from build123d import *

# Parameters (mm, degrees)
SKETCH1_R                = 143
SKETCH1_R_2              = 50
BOSS_EXTRUDE1_DEPTH      = 6.9
SKETCH2_R                = 1.85
BOSS_EXTRUDE2_DEPTH      = 6.9
FILLET1_R                = 30
CIRPATTERN1_COUNT        = 6
FILLET1_OF_CIRPATTERN1_R = 30
CUT_EXTRUDE1_DEPTH       = 214.214938645
FILLET3_R                = 5
CIRPATTERN2_COUNT        = 6
FILLET3_OF_CIRPATTERN2_R = 5
CUT_EXTRUDE2_DEPTH       = 10
FILLET4_R                = 10
FILLET5_START            = -1
FILLET5_DEPTH            = 9


with BuildPart() as part:
    # Sketch1 → Boss-Extrude1 (new body)
    with BuildSketch(Plane.XY):
        with Locations(Location((0, 0, 0), (0, 0, 180))):
            Circle(SKETCH1_R)
        with Locations(Location((0, 0, 0), (0, 0, 180))):
            Circle(SKETCH1_R_2, mode=Mode.SUBTRACT)
    extrude(amount=BOSS_EXTRUDE1_DEPTH)

    # Sketch2 → Boss-Extrude2 (add)
    with BuildSketch(Plane.XY.offset(6.9)):
        with BuildLine():
            Line((-136, -8), (-150, -8))
            ThreePointArc((-150, -8), (-158, 0), (-150, 8))
            Line((-150, 8), (-136, 8))
            ThreePointArc((-136, 8), (-128, 0), (-136, -8))
        make_face()
        with Locations((-150, 0)):
            Circle(SKETCH2_R, mode=Mode.SUBTRACT)
    boss_extrude2 = extrude(amount=-BOSS_EXTRUDE2_DEPTH)

    # Fillet1
    fillet1_edges = [part.edges().sort_by_distance(p)[0] for p in [
        (-142.776048411, 8, 3.45),
        (-142.776048411, -8, 3.45),
    ]]
    fillet(fillet1_edges, radius=FILLET1_R)

    # CirPattern1: Boss-Extrude2 ×6 about axis
    cirpattern1_axis = Axis((0, 0, 0), (0, 0, 1))
    for i in range(1, CIRPATTERN1_COUNT):
        add(boss_extrude2.rotate(cirpattern1_axis, i * 360 / CIRPATTERN1_COUNT))

    # Fillet1 of CirPattern1
    fillet1_of_cirpattern1_edges = [part.edges().sort_by_distance(p)[0] for p in [
        (-78.316227436, -119.647684976, 3.45),
        (-64.459820975, -127.647684976, 3.45),
        (64.459820975, -127.647684976, 3.45),
        (78.316227436, -119.647684976, 3.45),
        (142.776048411, -8, 3.45),
        (142.776048411, 8, 3.45),
        (78.316227436, 119.647684976, 3.45),
        (64.459820975, 127.647684976, 3.45),
        (-64.459820975, 127.647684976, 3.45),
        (-78.316227436, 119.647684976, 3.45),
    ]]
    fillet(fillet1_of_cirpattern1_edges, radius=FILLET1_OF_CIRPATTERN1_R)

    # Sketch7 → Cut-Extrude1 (cut, through all)
    with BuildSketch(Plane.XY.offset(6.9)):
        with BuildLine():
            Line((-30, 158), (30, 158))
            ThreePointArc((30, 158), (45, 143), (30, 128))
            Line((30, 128), (-30, 128))
            ThreePointArc((-30, 128), (-45, 143), (-30, 158))
        make_face()
    cut_extrude1 = extrude(amount=-CUT_EXTRUDE1_DEPTH, mode=Mode.SUBTRACT)

    # Fillet3
    fillet3_edges = [part.edges().sort_by_distance(p)[0] for p in [
        (43.398254251, 136.255610996, 3.45),
        (-43.398254251, 136.255610996, 3.45),
    ]]
    fillet(fillet3_edges, radius=FILLET3_R)

    # CirPattern2: Cut-Extrude1 ×6 about axis
    cirpattern2_axis = Axis((0, 0, 0), (0, 0, 1))
    for i in range(1, CIRPATTERN2_COUNT):
        add(cut_extrude1.rotate(cirpattern2_axis, i * 360 / CIRPATTERN2_COUNT), mode=Mode.SUBTRACT)

    # Fillet3 of CirPattern2
    fillet3_of_cirpattern2_edges = [part.edges().sort_by_distance(p)[0] for p in [
        (-96.301693406, 105.711796159, 3.45),
        (-139.699947656, 30.543814837, 3.45),
        (-139.699947656, -30.543814837, 3.45),
        (-96.301693406, -105.711796159, 3.45),
        (-43.398254251, -136.255610996, 3.45),
        (43.398254251, -136.255610996, 3.45),
        (96.301693406, -105.711796159, 3.45),
        (139.699947656, -30.543814837, 3.45),
        (139.699947656, 30.543814837, 3.45),
        (96.301693406, 105.711796159, 3.45),
    ]]
    fillet(fillet3_of_cirpattern2_edges, radius=FILLET3_OF_CIRPATTERN2_R)

    # Sketch8 → Cut-Extrude2 (cut)
    with BuildSketch(Plane.XY.offset(6.9)):
        with BuildLine():
            Line((88.826969439, -117.302003887), (84.326969439, -109.507775253))
            ThreePointArc((84.326969439, -109.507775253), (78.727650946, -108.125342861), (77.567379868, -113.774878941))
            Line((77.567379868, -113.774878941), (81.895896581, -121.29702529))
            ThreePointArc((81.895896581, -121.29702529), (87.360379041, -122.76754121), (88.826969439, -117.302003887))
        make_face()
        with BuildLine():
            Line((64.101233792, -131.577414018), (59.601233792, -123.783185384))
            ThreePointArc((59.601233792, -123.783185384), (54.136918717, -122.319207019), (52.673277073, -127.783612295))
            Line((52.673277073, -127.783612295), (57.221343973, -135.658853653))
            ThreePointArc((57.221343973, -135.658853653), (62.677994964, -137.017599926), (64.101233792, -131.577414018))
        make_face()
    extrude(amount=-CUT_EXTRUDE2_DEPTH, mode=Mode.SUBTRACT)

    # Fillet4
    fillet4_edges = [part.edges().sort_by_distance(p)[0] for p in [
        (64.565608345, -134.330457838, 3.45),
        (84.050784817, -123.080685956, 3.45),
    ]]
    fillet(fillet4_edges, radius=FILLET4_R)

    # Fillet5: read off the stored shape, not the designer's step
    # Fillet5 outline → Fillet5 (cut)
    with BuildSketch(Plane.XY.offset(FILLET5_START)):
        with BuildLine():
            ThreePointArc((87.553061033, -115.095529803), (90.213766815, -111.477504252), (93.384762884, -108.297213687))
            ThreePointArc((93.384762884, -108.297213687), (88.166794559, -109.665787745), (82.997135719, -108.124743986))
            ThreePointArc((82.997135719, -108.124743986), (83.746204288, -108.73534476), (84.326969439, -109.507775253))
            Line((84.326969439, -109.507775253), (87.553061033, -115.095529803))
        make_face()
        with BuildLine():
            ThreePointArc((52.14020721, -125.939999968), (50.889960833, -131.187577731), (47.09575677, -135.022183827))
            ThreePointArc((47.09575677, -135.022183827), (51.435909668, -133.866082974), (55.900021902, -133.370907928))
            Line((55.900021902, -133.370907928), (52.673277073, -127.783612295))
            ThreePointArc((52.673277073, -127.783612295), (52.294537166, -126.894249553), (52.14020721, -125.939999968))
        make_face()
    extrude(amount=FILLET5_DEPTH, mode=Mode.SUBTRACT)


solid = part.part
Build history of the part. All positions in model axes, mm. A direction names the side the tool comes from. Coordinates: 2 decimals unless noted, no trailing zeros. Order: outer loops, then holes, each group sorted by start corner. A loop starts at its lowest first (then second) coordinate and runs counter-clockwise, first axis right, second up. Notation, with made-up numbers: (4, 20) - (21, 20) arc R19 ccw to (21, 50) - close; hole circle Ø6 at (-34.5, 87). An arc over 180 degrees is marked (long way). Write each question's results on one line, items separated by ' | '. Start each with the question number.
Item 1: Band-saw the part on A-A on x = 0. Write the cut outline in (y, z).
Item 2: Mould opens along Y. For faces 4 (the face through (36.324, -129.398, 3.498)), 5 (the face through (-93.9, -96.16, 3.5)), 6 (the face through (2, 59, 0)) say: released by +Y, released by -Y, zero draft, split by the parting line, or undercut.
Item 3: Tool access for faces 1 (the face through (110.641, -64.364, 3.498)), 2 (the face through (36.492, 129.478, 3.498)), 3 (the face through (0, -128, 3)): list every direction of +Z, -Z, +X, -X, +Y, -Y with a clear straight run to the whole face (end or side of a thin tool).
Item 4: Flat gauge pins, fed straight in: pin 1 (1.5 mm diameter, centred on x = -56.5, z = 2.5, fed in from +Y); pin 2 (2 mm diameter, centred on x = -75, y = 129.9, fed in from +Z); pin 3 (3 mm diameter, centred on x = 59, z = 1.5, fed in from +Y); pin 4 (1.5 mm diameter, centred on x = -87, z = 2.5, fed in from -Y). Where does each tip first touch, or does it go through?
Item 5: Band-saw the part on C-C on y = -85. Write the cut outline in (x, z), and give its area (3 significant figures).
Item 6: Band-saw the part on D-D on x = 109.5. Write the cut outline in (y, z), and give its area (4 significant figures).
Item 7: Wall check: probe 1 along Y at (x, z) = (75, 3); probe 2 along Y at (x, z) = (0, 4.75); probe 3 along Y at (x, z) = (-150, 3.25). Give the ranges that are in metal, low to high. Write a range as [from, to].
Item 8: Band-saw the part on B-B on z = 2.25. State how many separate pieces and enclosed holes the cut face has, and give its area (3 significant figures).
Numbers:
1) outline: (-128, 0) - (-50, 0) - (-50, 6.9) - (-128, 6.9) - close; (50, 0) - (128, 0) - (128, 6.9) - (50, 6.9) - close
2) face 4: released by -Y | face 5: undercut | face 6: zero draft
3) face 1: +Z, -Z, +X, -Y | face 2: +Z, -Z, +Y | face 3: +Z, -Z, -Y
4) pin 1: y = 133.38 | pin 2: through | pin 3: y = 133.56 | pin 4: y = -117.4
5) outline: (-98.73, 0) - (98.73, 0) - (98.73, 6.9) - (-98.73, 6.9) - close | area: 1,360 mm^2
6) outline: (-66.34, 0) - (66.34, 0) - (66.34, 6.9) - (-66.34, 6.9) - close | area: 915.5 mm^2
7) probe 1: [-137.9, -131.75], [-128.05, 128.05], [131.75, 137.9] | probe 2: [-128, -50], [50, 128] | probe 3: [-9.94, -1.85], [1.85, 9.94]
8) separate pieces: 1 | enclosed holes: 7 | area: 51,700 mm^2
